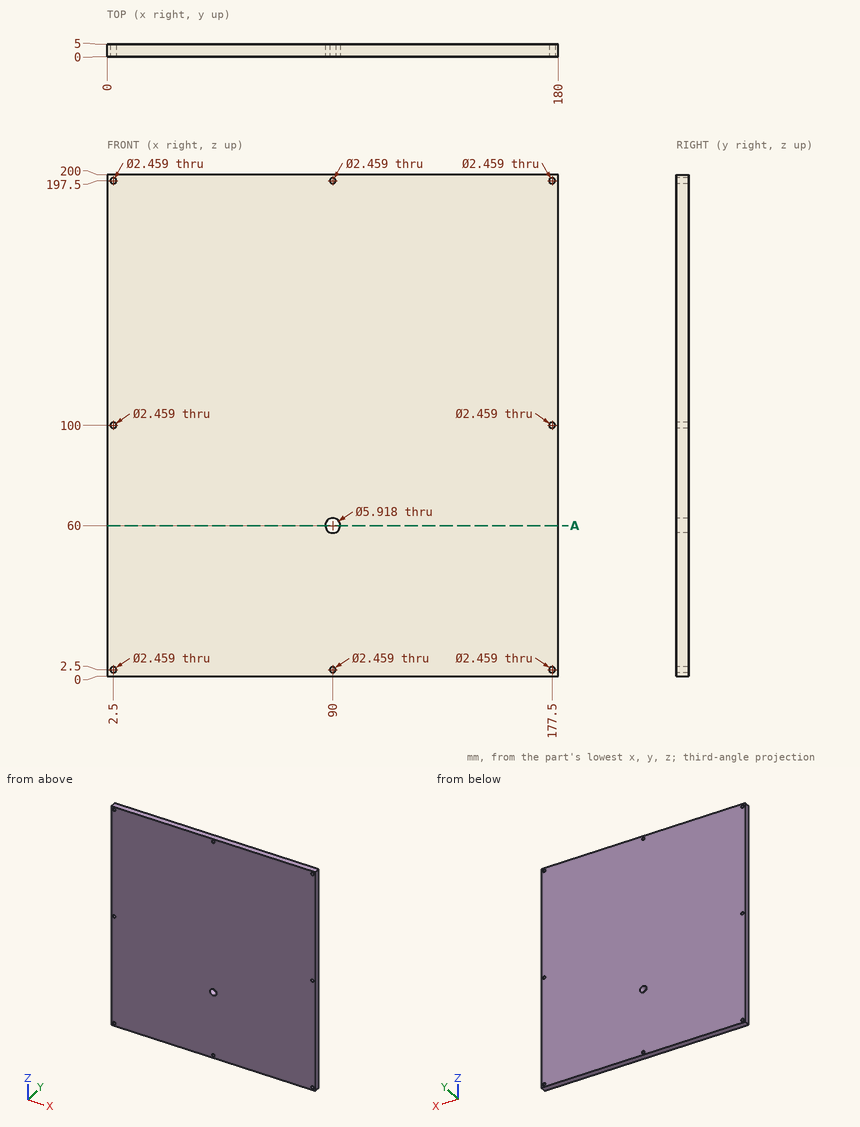
Design review of the part shown in the three views and the two pictorial views. Dimensions are in mm from the part's minimum x, y and z. Coordinates: 2 decimals unless noted, no trailing zeros. Loops run counter-clockwise (first coordinate to the right, second up) from the corner with the lowest first, then second, coordinate; pieces in that order, holes last. Notation, with made-up numbers: (40, -23) - (49, -23) arc R23 cw to (49, 7) - close; hole circle Ø9 at (88.5, -26.75). An arc over 180 degrees is marked (long way). Use a Markdown table: item, result. Add a question column.
Item 1: We need section A-A (z = 60). Give the boundary of the cut face in (x, y).
Item 2: Insertion check: pin 1 Ø3 at (x, z) = (177.5, 197.5) entering from -Y; pin 2 Ø2 at (x, z) = (177.5, 2.5) entering from +Y. Each pin has a flat end and moves straight along its axis. Give the tip position at first contact, or say it passes through.
Item 3: For line 1 (Z direction, x = 2.5, y = 3); line 2 (X direction, y = 2.25, z = 100); line 3 (X direction, y = 3.55, z = 197.5), list the stretches that pass through material, from the lowest coordinate up.
Results list:
| question | item | result |
|---|---|---|
| 1 | outline | (0, 0) - (87.04, 0) - (87.04, 5) - (0, 5) - close; (92.96, 0) - (180, 0) - (180, 5) - (92.96, 5) - close |
| 2 | pin 1 | stops at y = 0 |
| 2 | pin 2 | passes through |
| 3 | line 1 | z = 0 to 1.27, 3.73 to 98.77, 101.23 to 196.27, 198.73 to 200 |
| 3 | line 2 | x = 0 to 1.27, 3.73 to 176.27, 178.73 to 180 |
| 3 | line 3 | x = 0 to 1.27, 3.73 to 88.77, 91.23 to 176.27, 178.73 to 180 |
